Autodesk Inventor part; units mm, degrees
ref_plane "YZ Plane" through (0, 0, 0) normal (1, 0, 0) x (0, 1, 0)
ref_plane "XZ Plane" through (0, 0, 0) normal (0, 1, 0) x (-1, 0, 0)
ref_plane "XY Plane" through (0, 0, 0) normal (0, 0, 1) x (1, 0, 0)
sketch "Sketch1" plane through (0, 0, 0) normal (0, 1, 0) x (-1, 0, 0)
  line L0 (19, 19) -> (-19, 19)
  line L1 (-19, 19) -> (-19, -19)
  line L2 (-19, -19) -> (19, -19)
  line L3 (19, -19) -> (19, 19)
  line L4 (19, 19) -> (-19, -19) construction
  line L5 (-19, 19) -> (19, -19) construction
  point P0 (0, 0)
  dimension "d0" = 38
  dimension "d1" = 38
extrude "Extrusion1" add sketch "Sketch1" along normal blind 2
sketch "Sketch2" plane through (0, 2, 0) normal (0, 1, 0) x (1, 0, 0)
  line L0 (8.5, -12) -> (-8.5, -12)
  line L1 (-8.5, -12) -> (-8.5, 12)
  line L2 (-8.5, 12) -> (8.5, 12)
  line L3 (8.5, 12) -> (8.5, -12)
  line L4 (8.5, -12) -> (-8.5, 12) construction
  line L5 (-8.5, -12) -> (8.5, 12) construction
  point P0 (0, 0)
  dimension "d4" = 17
  dimension "d5" = 24
extrude "Extrusion2" add sketch "Sketch2" along normal blind 14.34
sketch "Sketch3" plane through (0, 16.34, 0) normal (0, 1, 0) x (1, 0, 0)
  circle A0 centre (0, 0) radius 8.45
  dimension "d8" = 16.9
extrude "Extrusion3" add sketch "Sketch3" along normal blind 17.7
sketch "Sketch4" plane through (0, 34.04, 0) normal (0, 1, 0) x (1, 0, 0)
  circle A0 centre (0, 0) radius 11
  dimension "d13" = 22
extrude "Extrusion4" add sketch "Sketch4" along normal blind 22
sketch "Sketch5" plane through (0, 56.04, 0) normal (0, 1, 0) x (1, 0, 0)
  circle A0 centre (0, 0) radius 13.45
  dimension "d16" = 26.9
extrude "Extrusion5" add sketch "Sketch5" along normal blind 8
properties part number "Camera"
Input: part model. Units: mm. Frame: model coordinates. A direction names the side the tool comes from. Coordinates: 2 decimals unless noted, no trailing zeros. Loops run counter-clockwise (first coordinate to the right, second up) from the corner with the lowest first, then second, coordinate; pieces in that order, holes last.
Q1. Contact query for flat-ended pins moving along their axis: pin 1 (11.5 mm diameter, centred on x = 4, y = 12.5, fed in from -Z); pin 2 (2 mm diameter, centred on y = 49.5, z = -8.5, fed in from +X); pin 3 (8 mm diameter, centred on x = -4.5, y = 13.5, fed in from +Z); pin 4 (3 mm diameter, centred on y = 35.5, z = 13, fed in from +X). Output: stop coordinate, or through.
Q2. Cut plane D-D (y = 12). Output: boundary loops of the cut face in (x, z), then the cut area to 3 significant figures.
Q3. Draft query along Y for faces 1 (the face through (0, 0, 0)), 2 (the face through (-4, 16.34, -8)), 3 (the face through (-19, 1, 0)). Return one class per face: +Y half, -Y half, draft (parallel to the pull), parting line (faces both ways), or undercut.
Q4. Cut plane A-A (x = 0). Output: boundary loops of the cut face in (y, z), then the cut area to 3 significant figures.
Q5. Cut plane C-C (z = 0). Output: boundary loops of the cut face in (x, y), then the cut area to 3 significant figures.
Q6. Cut plane B-B (z = -10). Output: boundary loops of the cut face in (x, y).
Q7. Material intervals for line 1 (Y direction, x = -12, z = 5.5); line 2 (Y direction, x = -5, z = -11.5); line 3 (Y direction, x = 7, z = 17.5), sorted ascending.
Q8. Set-up query: faces 4 (the face through (8.5, 9, 0)), 5 (the face through (0, 9, 12)), 6 (the face through (-8.5, 9, 0)), 7 (the face through (0, 9, -12)), 8 (the face through (9, 2, 0)). Return all of +Z, -Z, +X, -X, +Y, -Y with unobstructed straight access to the full face (end or side cutting, diameter ignored); none if empty.
Working result:
1. pin 1: stops at z = -12
1. pin 2: stops at x = 8.05
1. pin 3: stops at z = 12
1. pin 4: passes through
2. outline: (-8.5, -12) - (8.5, -12) - (8.5, 12) - (-8.5, 12) - close
2. area: 408 mm2
3. face 1: -Y half
3. face 2: undercut
3. face 3: draft
4. outline: (0, -19) - (2, -19) - (2, -12) - (16.34, -12) - (16.34, -8.45) - (34.04, -8.45) - (34.04, -11) - (56.04, -11) - (56.04, -13.45) - (64.04, -13.45) - (64.04, 13.45) - (56.04, 13.45) - (56.04, 11) - (34.04, 11) - (34.04, 8.45) - (16.34, 8.45) - (16.34, 12) - (2, 12) - (2, 19) - (0, 19) - close
4. area: 1,420 mm2
5. outline: (-19, 0) - (19, 0) - (19, 2) - (8.5, 2) - (8.5, 16.34) - (8.45, 16.34) - (8.45, 34.04) - (11, 34.04) - (11, 56.04) - (13.45, 56.04) - (13.45, 64.04) - (-13.45, 64.04) - (-13.45, 56.04) - (-11, 56.04) - (-11, 34.04) - (-8.45, 34.04) - (-8.45, 16.34) - (-8.5, 16.34) - (-8.5, 2) - (-19, 2) - close
5. area: 1,320 mm2
6. outline: (-19, 0) - (19, 0) - (19, 2) - (8.5, 2) - (8.5, 16.34) - (-8.5, 16.34) - (-8.5, 2) - (-19, 2) - close; (-8.99, 56.04) - (-4.58, 56.04) - (-4.58, 34.04) - (4.58, 34.04) - (4.58, 56.04) - (8.99, 56.04) - (8.99, 64.04) - (-8.99, 64.04) - close
7. line 1: y = 0 to 2, 56.04 to 64.04
7. line 2: y = 0 to 16.34, 56.04 to 64.04
7. line 3: y = 0 to 2
8. face 4: +Z, -Z, +X
8. face 5: +Z, +X, -X
8. face 6: +Z, -Z, -X
8. face 7: -Z, +X, -X
8. face 8: none
